Study the drawing (mm; zero at the part's minimum x, y, z) and answer. Round coordinates to 2 decimals unless told otherwise and drop trailing zeros. Write each loop counter-clockwise with the first axis right and the second up, starting at its lowest first coordinate (ties: lowest second). Pieces come first, ordered by that corner, then holes. Notation, with made-up numbers: (29, 82.5) -> (85, 82.5) arc R31 cw to (85, 111.5) -> close; hole circle Ø7 at (-4, 44). An arc over 180 degrees is marked (long way). One line per question, with ' | ' between items. Start each with the question number.
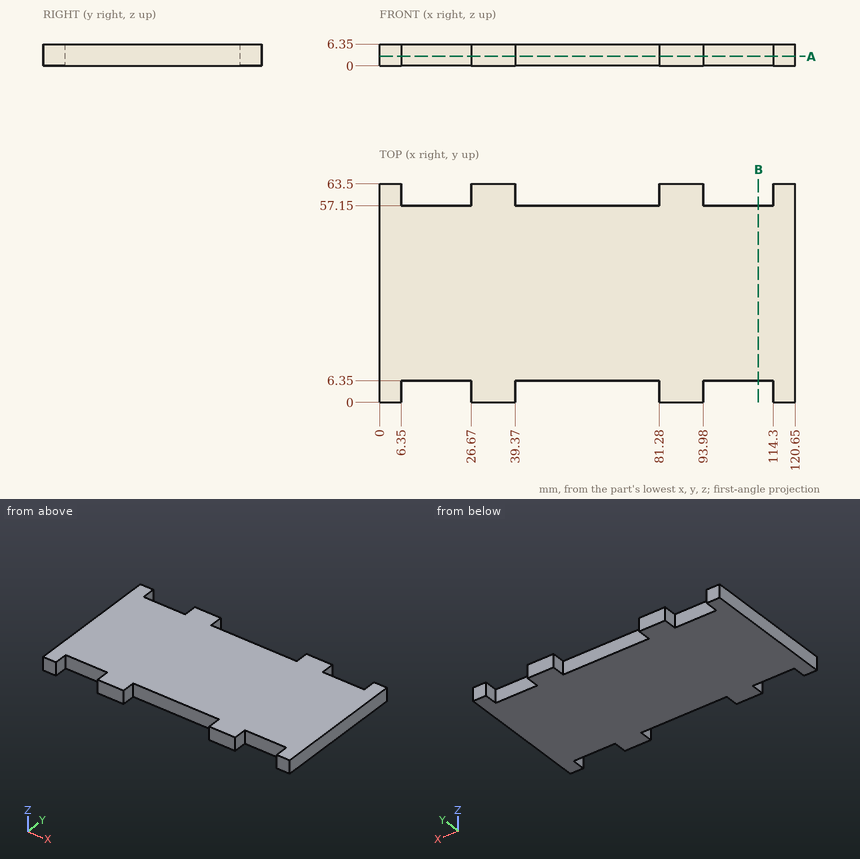
(1) Given pin 1 Ø3 at (x, z) = (100, 3.5) entering from -Y; pin 2 Ø3 at (x, z) = (58.5, 4) entering from +Y, each flat-ended and moving along its own axis, determine where each tip first touches the part or whether it passes through.
(2) A cutting plane is placed at B-B, the plane x = 110. Determine the outline of the cut face in (y, z).
(3) Consider L1, parallel to X at y = 57.5, z = 1.25; L2, parallel to Y at x = 47, z = 5.75. Determine where each line is inside the solid, lowest interval first.
(4) A cutting plane is placed at A-A, the plane z = 2.75. Determine the outline of the cut face in (x, y), then the cut area to 3 significant figures.
Returned:
1) pin 1: y = 6.35 | pin 2: y = 57.15
2) outline: (6.35, 0) -> (57.15, 0) -> (57.15, 6.35) -> (6.35, 6.35) -> close
3) L1: 0 to 6.35, 26.67 to 39.37, 81.28 to 93.98, 114.3 to 120.65 | L2: 6.35 to 57.15
4) outline: (0, 0) -> (6.35, 0) -> (6.35, 6.35) -> (26.67, 6.35) -> (26.67, 0) -> (39.37, 0) -> (39.37, 6.35) -> (81.28, 6.35) -> (81.28, 0) -> (93.98, 0) -> (93.98, 6.35) -> (114.3, 6.35) -> (114.3, 0) -> (120.65, 0) -> (120.65, 63.5) -> (114.3, 63.5) -> (114.3, 57.15) -> (93.98, 57.15) -> (93.98, 63.5) -> (81.28, 63.5) -> (81.28, 57.15) -> (39.37, 57.15) -> (39.37, 63.5) -> (26.67, 63.5) -> (26.67, 57.15) -> (6.35, 57.15) -> (6.35, 63.5) -> (0, 63.5) -> close | area: 6,610 mm2
